from build123d import *

# Parameters (mm, degrees)
SKETCH1_R           = 16.5
BOSS_EXTRUDE1_DEPTH = 15
SKETCH2_R           = 21
BOSS_EXTRUDE2_DEPTH = 6
SKETCH3_R           = 12
CUT_EXTRUDE1_DEPTH  = 37.373066959
CHAMFER1_SIZE       = 2.5
CHAMFER1_SIZE2      = 0.669872981


with BuildPart() as part:
    # Sketch1 → Boss-Extrude1 (new body)
    with BuildSketch(Plane(origin=(0, 0, 0), x_dir=(1, 0, 0), z_dir=(0, 1, 0))):
        with Locations(Location((0, 0, 0), (0, 0, 270))):
            Circle(SKETCH1_R)
    extrude(amount=BOSS_EXTRUDE1_DEPTH)

    # Sketch2 → Boss-Extrude2 (add)
    with BuildSketch(Plane(origin=(0, 15, 0), x_dir=(1, 0, 0), z_dir=(0, 1, 0))):
        with Locations(Location((0, 0, 0), (0, 0, 270))):
            Circle(SKETCH2_R)
    extrude(amount=BOSS_EXTRUDE2_DEPTH)

    # Sketch3 → Cut-Extrude1 (cut, through all)
    with BuildSketch(Plane(origin=(0, 21, 0), x_dir=(1, 0, 0), z_dir=(0, 1, 0))):
        with Locations(Location((0, 0, 0), (0, 0, 270))):
            Circle(SKETCH3_R)
    extrude(amount=-CUT_EXTRUDE1_DEPTH, mode=Mode.SUBTRACT)

    # Chamfer1
    chamfer1_edges = [part.edges().sort_by_distance(p)[0] for p in [
        (0, 21, -12),
    ]]
    chamfer1_side = [part.faces().sort_by_distance(p)[0] for p in [
        (0, 21, -20.406030304),
    ]]
    chamfer(chamfer1_edges, length=CHAMFER1_SIZE, length2=CHAMFER1_SIZE2, reference=chamfer1_side[0])


solid = part.part
Verification items for the finished model (mm, model axes). A direction names the side the tool comes from. Coordinates: 2 decimals unless noted, no trailing zeros. Write each loop counter-clockwise with the first axis right and the second up, starting at its lowest first coordinate (ties: lowest second). Pieces come first, ordered by that corner, then holes. Notation, with made-up numbers: (41, -24.5) -> (81, -24.5) arc R22 cw to (81, -6.5) -> close; hole circle Ø4 at (39.5, -16). An arc over 180 degrees is marked (long way). One line per item, written item: value. Start each with the question number.
Q1. Cross-section at D-D on z = 15.5. Enter the section's corners in (x, y), and give its area (3 significant figures).
Q2. Mould release check, pull along Z, two halves, no side actions. Record for faces 3 (the cylindrical face through (6.31, 17.96, 20.03)), 4 (the flat face through (-14, 21, -5)), 5 (the cylindrical face through (3.604, 10.307, 11.446)): pulls with the +Z half, pulls with the -Z half, needs draft (parallel to the pull), parting line crosses it, or undercut.
Q3. Access from +Z, -Z, +X, -X, +Y, -Y to the whole of each face (thin tool, end or side, straight path). Record for faces 1 (the flat face through (-12.15, 0, 1.15)), 2 (the flat face through (-11, 15, -13)).
Q4. Cross-section at C-C on y = 19.5. Enter the section's corners in (x, z), and give its area (3 significant figures).
Q5. Thickness scan on L1, parallel to X at y = 5.25, z = 0; L2, parallel to X at y = 17.25, z = 0; L3, parallel to Z at x = -5, y = 8.5. Record the ranges inside material, lowest first. Write a range as from..to.
Q6. Go/stop test with flat-tipped pins: P1, Ø5, axis at x = -16, y = 3, coming from the -Z side; P2, Ø10, axis at y = 15.5, z = -7.5, coming from the -X side; P3, Ø5, axis at x = -8, z = 8.5, coming from the +Y side. Record where each tip stops, or that it passes through.
Q7. Cross-section at B-B on z = 0. Enter the section's corners in (x, y).
Q8. Cross-section at A-A on x = 0. Enter the section's corners in (y, z), and give its area (3 significant figures).
Checked values:
1. outline: (-14.17, 15) -> (-5.66, 15) -> (-5.66, 0) -> (5.66, 0) -> (5.66, 15) -> (14.17, 15) -> (14.17, 21) -> (-14.17, 21) -> close
1. area: 340 mm²
2. face 3: parting line crosses it
2. face 4: needs draft
2. face 5: undercut
3. face 1: +Z, -Z, +X, -X, -Y
3. face 2: -Y
4. outline: circle Ø42 at (0, 0); hole circle Ø24 at (0, 0)
4. area: 933 mm²
5. L1: x = -16.5..-12, 12..16.5
5. L2: x = -21..-12, 12..21
5. L3: z = -15.72..-10.91, 10.91..15.72
6. P1: stops at z = -9.49
6. P2: stops at x = -20.85
6. P3: stops at y = 20.91
7. outline: (-21, 15) -> (-16.5, 15) -> (-16.5, 0) -> (-12, 0) -> (-12, 20.33) -> (-14.5, 21) -> (-21, 21) -> close; (12, 0) -> (16.5, 0) -> (16.5, 15) -> (21, 15) -> (21, 21) -> (14.5, 21) -> (12, 20.33) -> close
8. outline: (0, -16.5) -> (15, -16.5) -> (15, -21) -> (21, -21) -> (21, -14.5) -> (20.33, -12) -> (0, -12) -> close; (0, 12) -> (20.33, 12) -> (21, 14.5) -> (21, 21) -> (15, 21) -> (15, 16.5) -> (0, 16.5) -> close
8. area: 241 mm²
